from build123d import *

# Parameters (mm, degrees)
F0_W     = 1524
F0_H     = 152.4
F0_W_2   = 1485.9
F0_H_2   = 114.3
F1_DEPTH = 1828.8
F2_W     = 114.3
F2_H     = 317.5
F3_DEPTH = 25.4
F5_DEPTH = 25.4
F7_DEPTH = 25.4


with BuildPart() as f1:
    # F0 (on Top) → F1 (new body)
    with BuildSketch(Plane.XY):
        Rectangle(F0_W, F0_H)
        Rectangle(F0_W_2, F0_H_2, mode=Mode.SUBTRACT)
    extrude(amount=F1_DEPTH)

    # F2 (on face) → F3 (cut)
    with BuildSketch(Plane.YZ.offset(762)):
        with Locations((0, 158.75)):
            Rectangle(F2_W, F2_H)
    extrude(amount=-F3_DEPTH, mode=Mode.SUBTRACT)

    # F4 (on face) → F5 (cut)
    with BuildSketch(Plane(origin=(0, 76.2, 0), x_dir=(-1, 0, 0), z_dir=(0, 1, 0))):
        with BuildLine():
            ThreePointArc((38.1, 1320.8), (26.940768, 1347.740768), (0, 1358.9))
            ThreePointArc((0, 1358.9), (-26.940768, 1293.859232), (38.1, 1320.8))
        make_face()
        with BuildLine():
            ThreePointArc((38.1, 450.85), (-26.940768, 477.790768), (0, 412.75))
            ThreePointArc((0, 412.75), (26.940768, 423.909232), (38.1, 450.85))
        make_face()
    extrude(amount=-F5_DEPTH, mode=Mode.SUBTRACT)

    # F6 (on face) → F7 (cut)
    with BuildSketch(Plane.XZ.offset(76.2)):
        with BuildLine():
            ThreePointArc((38.1, 1320.8), (26.940768, 1347.740768), (0, 1358.9))
            ThreePointArc((0, 1358.9), (-26.940768, 1293.859232), (38.1, 1320.8))
        make_face()
        with BuildLine():
            ThreePointArc((38.1, 450.85), (-26.940768, 477.790768), (0, 412.75))
            ThreePointArc((0, 412.75), (26.940768, 423.909232), (38.1, 450.85))
        make_face()
    extrude(amount=-F7_DEPTH, mode=Mode.SUBTRACT)


solid = f1.part
Geometry: final body of the model. Coordinates: model frame, mm. A direction names the side the tool comes from. Give positions to 0.01 mm unless a question says otherwise; leave off trailing zeros. Loops run counter-clockwise (first coordinate to the right, second up) from the corner with the lowest first, then second, coordinate; pieces in that order, holes last. Notation, with made-up numbers: M 43.25,53 L 82.25,53 A24 cw 82.25,65 Z; hole C 24.5,18 d3. An arc over 180 degrees is marked long. Put each result on its own line as item: value. Start each with the question number.
1) Pull-direction query (Y, two-part tool) for faces 1 (the flat face through (742.95, -1, 1063)), 2 (the flat face through (-11, 76.2, 902)), 3 (the flat face through (-4, 62, 1828.8)); classes: pulls with the +Y half, pulls with the -Y half, needs draft (parallel to the pull), parting line crosses it, or undercut.
2) Access query for faces 4 (the flat face through (-742.95, -1, 902)), 5 (the flat face through (-762, -1, 902)). Directions: +Z, -Z, +X, -X, +Y, -Y. A direction counts if a zero-diameter tool reaches every point of the face in a straight line with its end or side. Return the directions, or none.
3) Ray query, line 1 along Y through (x, z) = (628, 1479); line 2 along Z through (x, y) = (0, -71.5); line 3 along X through (y, z) = (-70.5, 1320.8). Return the intervals inside material, ascending.
4) Cut plane B-B (y = 36.5). Output: boundary loops of the cut face in (x, z).
5) Contact query for flat-ended pins moving along their axis: pin 1 (1.5 mm diameter, centred on y = 49, z = 286.5, fed in from +X); pin 2 (5.5 mm diameter, centred on x = 753.5, y = -24, fed in from -Z). Output: stop coordinate, or through.
6) Cut plane C-C (z = 930). Output: boundary loops of the cut face in (x, y), then the cut area to 3 significant figures.
7) Cut plane A-A (x = -351.5). Output: boundary loops of the cut face in (y, z), then the cut area to 3 significant figures.
Verdict:
1. face 1: undercut
1. face 2: pulls with the +Y half
1. face 3: needs draft
2. face 4: +Z, -Z
2. face 5: +Z, -Z, -X, +Y, -Y
3. line 1: -76.2 to -57.15, 57.15 to 76.2
3. line 2: 0 to 412.75, 488.95 to 1282.7, 1358.9 to 1828.8
3. line 3: -762 to -38.1, 38.1 to 762
4. outline: M -762,0 L -742.95,0 L -742.95,1828.8 L -762,1828.8 Z; M 742.95,317.5 L 762,317.5 L 762,1828.8 L 742.95,1828.8 Z
5. pin 1: x = -742.95
5. pin 2: z = 317.5
6. outline: M -762,-76.2 L 762,-76.2 L 762,76.2 L -762,76.2 Z; hole M -742.95,-57.15 L 742.95,-57.15 L 742.95,57.15 L -742.95,57.15 Z
6. area: 62,400 mm2
7. outline: M -76.2,0 L -57.15,0 L -57.15,1828.8 L -76.2,1828.8 Z; M 57.15,0 L 76.2,0 L 76.2,1828.8 L 57.15,1828.8 Z
7. area: 69,700 mm2
